The listing builds one solid part. Answer for the finished solid, in the listing's coordinates (mm). A direction names the side the tool comes from. Give positions to 0.01 mm unless a question says otherwise; leave off trailing zeros. Write each loop counter-clockwise with the first axis right and the second up, starting at its lowest first coordinate (ties: lowest second). Pieces come first, ordered by that corner, then holes. Notation, with made-up numbers: (70.25, -39.5) - (74.25, -39.5) arc R20 ccw to (74.25, -34.5) - close; hole circle Ø5 at (-38, 21). An arc over 180 degrees is marked (long way). Return JSON: item names as keys, results as strings.
from build123d import *

# Parameters (mm, degrees)
F1_DEPTH = 4.7625
F2_R     = 9.525
F3_DEPTH = 4.7635
F4_SIZE  = 2.38124


# Not quite as in the source:
# - a fillet or chamfer is up to 0.001 mm smaller than in the source, because OpenCascade refuses the exact size
# - a feature of the source that left no trace in its solid (it failed there, or was rolled back) is left out


with BuildPart() as f1:
    # F0 (on Top) → F1 (new body)
    with BuildSketch(Plane.XY):
        Polygon((-3.074264621, 21.805118867), (-40.0660246394, 41.4531760826), (-21.6879004002, 3.8143528936), (-51.8053957451, -25.295317935), (-10.3295949709, -19.4477191337), (8.0485292683, -57.0865423226), (15.3038596181, -15.8337043219), (56.7796603923, -9.9861055206), (19.787900374, 9.6619516949), (27.0432307238, 50.9147896956), align=None)
    extrude(amount=F1_DEPTH)

    # F2 (on Top) → F3 (cut, through all)
    with BuildSketch(Plane.XY):
        with Locations((15.3038596181, -15.8337043219)):
            Circle(F2_R)
        with Locations((-10.3295949709, -19.4477191337)):
            Circle(F2_R)
        with Locations((-21.6879004002, 3.8143528936)):
            Circle(F2_R)
        with Locations((-3.074264621, 21.805118867)):
            Circle(F2_R)
        with Locations((19.787900374, 9.6619516949)):
            Circle(F2_R)
    extrude(amount=F3_DEPTH, mode=Mode.SUBTRACT)

    # F4 (size 2.38125 in the source; OpenCascade refuses exactly that, so slightly less here)
    f4_edges = [f1.edges().sort_by_distance(p)[0] for p in [
        (24.240507, 34.97888, 4.7625),
        (15.408887, 39.669767, 4.7625),
        (-1.744503, 12.373398, 4.7625),
        (-25.776163, 33.863161, 4.7625),
        (-32.966583, 26.913355, 4.7625),
        (-12.306882, 2.164469, 4.7625),
        (-40.171052, -14.050296, 4.7625),
        (-35.783356, -23.036399, 4.7625),
        (-5.861568, -11.035682, 4.7625),
        (0.949087, -42.546721, 4.7625),
        (10.851253, -41.150633, 4.7625),
        (8.684234, -8.984896, 4.7625),
        (40.75762, -12.245024, 4.7625),
        (42.489799, -2.39609, 4.7625),
        (11.22872, 5.482711, 4.7625),
        (24.240507, 34.97888, 0),
        (15.408887, 39.669767, 0),
        (-1.744503, 12.373398, 0),
        (-25.776163, 33.863161, 0),
        (-32.966583, 26.913355, 0),
        (-12.306882, 2.164469, 0),
        (-40.171052, -14.050296, 0),
        (-35.783356, -23.036399, 0),
        (-5.861568, -11.035682, 0),
        (0.949087, -42.546721, 0),
        (10.851253, -41.150633, 0),
        (8.684234, -8.984896, 0),
        (40.75762, -12.245024, 0),
        (42.489799, -2.39609, 0),
        (11.22872, 5.482711, 0),
    ]]
    chamfer(f4_edges, length=F4_SIZE)


solid = f1.part
Item 1: Consider L1, parallel to Y at x = -22, z = 1.2; L2, parallel to X at y = 23, z = 1; L3, parallel to Y at x = 16.5, z = 0.6. Determine where each line is inside the solid, lowest interval first.
Answer below:
{"L1": "y = -19.9 to -6.89, 14.52 to 30.52", "L2": "x = -29.52 to -13.91, 7.77 to 20.73", "L3": "y = -4.59 to -1.16, 20.48 to 38.25"}
Item 2: The mould has two halves that part along Y. Classify faces 1 (the face through (-36.2, -21.9, 1.2)), 2 (the face through (-2.019, 12.189, 2.232)), 3 (the face through (42.12, -3.57, 3.59)): +Y half, -Y half, draft (parallel to the pull), parting line (faces both ways), or undercut.
Answer below:
{"face 1": "-Y half", "face 2": "undercut", "face 3": "+Y half"}
Item 3: A cutting plane is placed at A-A on z = 1.35. Determine the outline of the cut face in (x, y), then the cut area to 3 significant figures.
Answer below:
{"outline": "(-48.81, -23.83) - (-20.88, -19.89) arc R10.56 cw (long way) to (-4.79, -28.44) - (7.58, -53.78) - (12.47, -26) arc R10.56 cw (long way) to (25.56, -13.35) - (53.49, -9.41) - (28.58, 3.82) arc R10.56 cw (long way) to (20.59, 20.19) - (25.48, 47.97) - (5.2, 28.36) arc R10.56 cw (long way) to (-12.84, 25.82) - (-37.75, 39.05) - (-25.37, 13.71) arc R10.56 cw (long way) to (-28.53, -4.23) - close", "area": "2,200 mm²"}
Item 4: For faces 4 (the face through (8.4, -9.1, 2.5)), 5 (the face through (-30.43, 24.4, 3.56)), 6 (the face through (23.01, 34.96, 3.59)), determine the directions among +Z, -Z, +X, -X, +Y, -Y from which every point of the face is accessible in a straight line to the end or side of a thin tool.
Answer below:
{"face 4": "+Z", "face 5": "+Z, -X", "face 6": "+Z, +X"}
Item 5: Flat-ended cylindrical pins translate along their axes: P1, Ø15, axis at x = -21.69, y = 3.81, coming from the -Z side; P2, Ø1, axis at x = -4, z = 3.5, coming from the +Y side. Find the tip coordinate at first contact, or state that the pin passes through.
Answer below:
{"P1": "passes through", "P2": "stops at y = 11.71"}
